```python
from build123d import *

# Parameters (mm, degrees)
SKETCH1_R               = 2
BOSS_EXTRUDE1_DEPTH     = 20
CUT_EXTRUDE1_DEPTH      = 21.199009877
CUT_EXTRUDE1_DEPTH_BACK = 21.199009877
SKETCH2_R               = 1


with BuildPart() as part:
    # Sketch1 → Boss-Extrude1 (new body)
    with BuildSketch(Plane(origin=(0, 0, 0), x_dir=(0, 0, -1), z_dir=(1, 0, 0))):
        Circle(SKETCH1_R)
    extrude(amount=-BOSS_EXTRUDE1_DEPTH)

    # Sketch2 → Cut-Extrude1 (cut, two sides: drawn at the far end of the back side and taken through both)
    with BuildSketch(Plane.XY.offset(-CUT_EXTRUDE1_DEPTH_BACK)):
        with Locations((-16, 0)):
            Circle(SKETCH2_R)
    extrude(amount=CUT_EXTRUDE1_DEPTH + CUT_EXTRUDE1_DEPTH_BACK, mode=Mode.SUBTRACT)

    # Sketch3 → Revolve1 (revolve)
    with BuildSketch(Plane(origin=(0, 0, 0), x_dir=(1, 0, 0), z_dir=(0, 1, 0))):
        with BuildLine():
            Line((2.757385023, 0), (0, 0))
            Line((0, 0), (0, 3.5))
            ThreePointArc((0, 3.5), (1.985229955, 2.227844932), (2.757385023, 0))
        make_face()
    revolve(axis=Axis((-7.558889504, 0, 0), (1, 0, 0)))


solid = part.part
```
Here's how the part is built. I have some questions about the finished solid (model axes, mm). Round coordinates to 2 decimals unless told otherwise and drop trailing zeros. Order: outer loops, then holes, each group sorted by start corner. A loop starts at its lowest first (then second) coordinate and runs counter-clockwise, first axis right, second up. Notation, with made-up numbers: M -3,74 L 44,74 A16 ccw 44,86 Z; hole C -2.75,33 d4. An arc over 180 degrees is marked long. Answer as CSV lines item,"result".
Item 1: Imagine slicing it at D-D on y = 1.5. List the corners of the cut face in (x, z) for me.
From the geometry:
outline,"M -20,-1.32 L 0,-1.32 L 0,-3.16 A3.27 ccw 0,3.16 L 0,1.32 L -20,1.32 Z"
Item 2: Imagine slicing it at A-A on y = 0. List the corners of the cut face in (x, z) for me, and give its area (3 significant figures).
From the geometry:
outline,"M -20,-2 L -17,-2 L -17,2 L -20,2 Z; M -15,-2 L 0,-2 L 0,-3.5 A3.6 ccw 0,3.5 L 0,2 L -15,2 Z"
area,"86.3 mm2"
Item 3: Imagine slicing it at B-B on z = 0. List the corners of the cut face in (x, y) for me, and give its area (3 significant figures).
From the geometry:
outline,"M -20,-2 L 0,-2 L 0,-3.5 A3.6 ccw 0,3.5 L 0,2 L -20,2 Z; hole C -16,0 d2"
area,"91.2 mm2"
Item 4: We'd pull the mould along X, two halves only. Please class faces 1 (the cylindrical face through (-10, 0, 2)), 2 (the cylindrical face through (-15.46, 0.84, -0.03)), 3 (the flat face through (0, -2, 2)): +X half, -X half, draft (parallel to the pull), parting line (faces both ways), or undercut.
From the geometry:
face 1,"draft"
face 2,"undercut"
face 3,"-X half"
Item 5: For pin 1 (4 mm diameter, centred on y = -2, z = -1, fed in from +X); pin 2 (2 mm diameter, centred on x = -7, z = 1.5, fed in from -Y); pin 3 (1.5 mm diameter, centred on x = -6.5, z = 2.5, fed in from +Y), each with a flat end and sliding along its axis, tell me the tip position at first contact or that it passes through.
From the geometry:
pin 1,"x = 2.75"
pin 2,"y = -1.94"
pin 3,"y = 0.97"
Item 6: Please list where these lines run through material, in increasing order: L1, parallel to Y at x = -16, z = -0.1; L2, parallel to X at y = 0, z = 0.05; L3, parallel to Y at x = -16, z = -0.7. Write a range as [from, to].
From the geometry:
L1,"[-2, -1], [1, 2]"
L2,"[-20, -17], [-15, 2.76]"
L3,"[-1.87, -1], [1, 1.87]"
Item 7: Imagine slicing it at C-C on x = -4.25. List the corners of the cut face in (y, z) for me.
From the geometry:
outline,"C 0,0 d4"
